Could you check a few things on this model? Use its own coordinates, in mm. Give positions to 0.01 mm unless a question says otherwise; leave off trailing zeros. Loops run counter-clockwise (first coordinate to the right, second up) from the corner with the lowest first, then second, coordinate; pieces in that order, holes last. Notation, with made-up numbers: (17.5, 39.5) -> (48.5, 39.5) arc R16 cw to (48.5, 66.5) -> close; hole circle Ø5 at (55, -39.75). An arc over 180 degrees is marked (long way). Write item = value, one per line. Start each with the question number.
1) I'm going to push flat-ended pins straight in: pin 1 Ø0.8 at (x, z) = (42, 0.5) entering from -Y; pin 2 Ø0.5 at (x, z) = (-45, 0.5) entering from +Y. Where does each tip first touch, or does it pass through?
2) I need wall thicknesses on probe 1 along X at (y, z) = (2, 0.2); probe 2 along X at (y, z) = (-7.75, -0.25); probe 3 along X at (y, z) = (4.75, 0.3). Which ranges of each line are inside material? Lowest first, please. Write a range as from..to.
3) I want a section at B-B (z = 0.2). Count the separate pieces of the cut face and the enclosed holes in it, and give its area (3 significant figures).
4) I want a section at C-C (x = 25). List the corners of the cut face in (y, z) for me, and give its area (3 significant figures).
5) I want a section at A-A (y = -3). List the corners of the cut face in (x, z) for me.
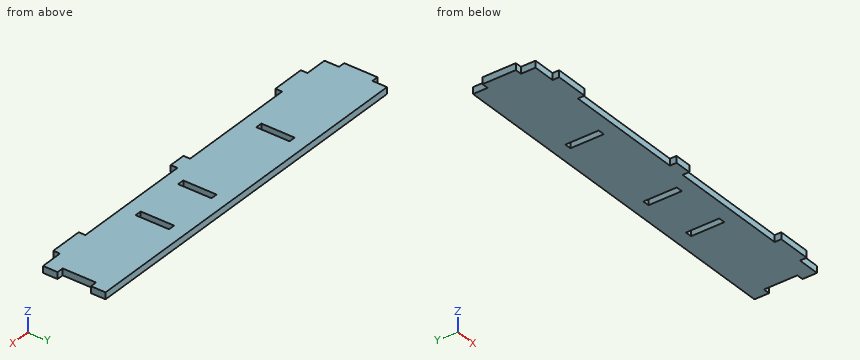
Autodesk Inventor part; units mm, degrees
ref_plane "YZ Plane" through (0, 0, 0) normal (1, 0, 0) x (0, 1, 0)
ref_plane "XZ Plane" through (0, 0, 0) normal (0, 1, 0) x (-1, 0, 0)
ref_plane "XY Plane" through (0, 0, 0) normal (0, 0, 1) x (1, 0, 0)
sketch "Sketch1" plane through (0, 0, 0) normal (0, 0, 1) x (1, 0, 0)
  line L0 (-62.09, 0) -> (62.09, 0) construction
  line L1 (0, 10.5) -> (0, -10.5) construction
  line L2 (44.35, -7.5) -> (-44.35, -7.5)
  line L3 (-44.35, -7.5) -> (-44.35, 7.5)
  line L4 (-44.35, 7.5) -> (44.35, 7.5)
  line L5 (44.35, 7.5) -> (44.35, -7.5)
  line L6 (44.35, -7.5) -> (-44.35, 7.5) construction
  line L7 (-44.35, -7.5) -> (44.35, 7.5) construction
  point P0 (0, 0)
  dimension "d0" = 88.7
  dimension "d1" = 15
extrude "Extrusion1" add sketch "Sketch1" along normal mid plane 1.6
sketch "Esquisse2" plane through (0, 0, 0.8) normal (0, 0, 1) x (1, 0, 0)
  line L0 (-44.35, -7.5) -> (44.35, -7.5) construction
  line L1 (44.35, -7.5) -> (44.35, 7.5) construction
  line L2 (44.35, 7.5) -> (-44.35, 7.5) construction
  line L3 (-44.35, 7.5) -> (-44.35, -7.5) construction
  line L4 (0, 10.82) -> (0, -12.42) construction
  line L5 (-62.09, 0) -> (62.09, 0) construction
  line L6 (-39, -7.5) -> (-31, -7.5)
  line L7 (-31, -7.5) -> (-31, -9.1)
  line L8 (-31, -9.1) -> (-39, -9.1)
  line L9 (-39, -9.1) -> (-39, -7.5)
  line L10 (31, -7.5) -> (39, -7.5)
  line L11 (39, -7.5) -> (39, -9.1)
  line L12 (39, -9.1) -> (31, -9.1)
  line L13 (31, -9.1) -> (31, -7.5)
  line L14 (-2, -7.5) -> (2, -7.5)
  line L15 (2, -7.5) -> (2, -9.1)
  line L16 (2, -9.1) -> (-2, -9.1)
  line L17 (-2, -9.1) -> (-2, -7.5)
  point P0 (0, 0)
  dimension "d4" = 8
  dimension "d5" = 1.6
  dimension "d8" = 70
  dimension "d13" = 4
  dimension "d14" = 1.6
extrude "Extrusion2" add sketch "Esquisse2" against normal blind 1.6
sketch "Esquisse3" plane through (0, 0, 0.8) normal (0, 0, 1) x (1, 0, 0)
  line L0 (-44.35, -7.5) -> (-39, -7.5) construction
  line L1 (-39, -9.1) -> (-39, -7.5) construction
  line L2 (-31, -9.1) -> (-39, -9.1) construction
  line L3 (-31, -7.5) -> (-31, -9.1) construction
  line L4 (-31, -7.5) -> (-2, -7.5) construction
  line L5 (-2, -9.1) -> (-2, -7.5) construction
  line L6 (2, -9.1) -> (-2, -9.1) construction
  line L7 (2, -7.5) -> (2, -9.1) construction
  line L8 (2, -7.5) -> (31, -7.5) construction
  line L9 (31, -9.1) -> (31, -7.5) construction
  line L10 (39, -9.1) -> (31, -9.1) construction
  line L11 (39, -7.5) -> (39, -9.1) construction
  line L12 (39, -7.5) -> (44.35, -7.5) construction
  line L13 (44.35, -7.5) -> (44.35, 7.5) construction
  line L14 (44.35, 7.5) -> (-44.35, 7.5) construction
  line L15 (-44.35, 7.5) -> (-44.35, -7.5) construction
  line L16 (0, 10.82) -> (0, -12.42) construction
  line L17 (-64.01, 0) -> (62.41, 0) construction
  line L18 (-44.35, 4) -> (-45.95, 4)
  line L19 (-45.95, 4) -> (-45.95, -4)
  line L20 (-45.95, -4) -> (-44.35, -4)
  line L21 (-44.35, -4) -> (-44.35, 4)
  point P0 (0, 0)
  dimension "d17" = 1.6
  dimension "d18" = 8
extrude "Extrusion3" add sketch "Esquisse3" against normal blind 1.6
sketch "Esquisse4" plane through (0, 0, 0.8) normal (0, 0, 1) x (1, 0, 0)
  line L0 (-18.25, -4) -> (-19.85, -4)
  line L1 (-19.85, -4) -> (-19.85, 4)
  line L2 (-19.85, 4) -> (-18.25, 4)
  line L3 (-18.25, 4) -> (-18.25, -4)
  line L4 (6.35, -4) -> (4.75, -4)
  line L5 (4.75, -4) -> (4.75, 4)
  line L6 (4.75, 4) -> (6.35, 4)
  line L7 (6.35, 4) -> (6.35, -4)
  line L8 (19.75, -4) -> (18.15, -4)
  line L9 (18.15, -4) -> (18.15, 4)
  line L10 (18.15, 4) -> (19.75, 4)
  line L11 (19.75, 4) -> (19.75, -4)
  line L12 (44.35, -4) -> (42.75, -4)
  line L13 (42.75, -4) -> (42.75, 4)
  line L14 (42.75, 4) -> (44.35, 4)
  line L15 (44.35, 4) -> (44.35, -4)
  point P0 (0, 0)
extrude "Extrusion4" cut sketch "Esquisse4" against normal blind 1.6
properties part number "FixationBatterieLateral" material "PVC-U"
Answer list:
q1.pin_1 = -7.5
q1.pin_2 = 4
q2.probe_1 = -45.95..-19.85, -18.25..4.75, 6.35..18.15, 19.75..42.75
q2.probe_2 = -39..-31, -2..2, 31..39
q2.probe_3 = -44.35..44.35
q3.separate_pieces = 1
q3.enclosed_holes = 3
q3.area = 1,320 mm^2
q4.outline = (-7.5, -0.8) -> (7.5, -0.8) -> (7.5, 0.8) -> (-7.5, 0.8) -> close
q4.area = 24.0 mm^2
q5.outline = (-45.95, -0.8) -> (-19.85, -0.8) -> (-19.85, 0.8) -> (-45.95, 0.8) -> close; (-18.25, -0.8) -> (4.75, -0.8) -> (4.75, 0.8) -> (-18.25, 0.8) -> close; (6.35, -0.8) -> (18.15, -0.8) -> (18.15, 0.8) -> (6.35, 0.8) -> close; (19.75, -0.8) -> (42.75, -0.8) -> (42.75, 0.8) -> (19.75, 0.8) -> close
